Design review of the part built by this model. Coordinates are the model's own, in mm. Coordinates: 2 decimals unless noted, no trailing zeros. Write each loop counter-clockwise with the first axis right and the second up, starting at its lowest first coordinate (ties: lowest second). Pieces come first, ordered by that corner, then holes. Notation, with made-up numbers: (6.5, -24.75) - (28.5, -24.75) arc R29 ccw to (28.5, 13.25) - close; hole circle Ø3 at (79, 51.5). An arc over 180 degrees is marked (long way). One line per item, written item: value.
from build123d import *

# Parameters (mm, degrees)
EXTRUDE_THIN1_DEPTH = 0.53
SKETCH2_R           = 1.151524856
CUT_EXTRUDE1_DEPTH  = 16.607776908


with BuildPart() as part:
    # Sketch1 → Extrude-Thin1 (new body)
    with BuildSketch(Plane(origin=(0, 0, 0), x_dir=(1, 0, 0), z_dir=(0, 1, 0))):
        with BuildLine():
            ThreePointArc((9.712852175, 5.226987912), (-10.721135618, -2.591939635), (11.027949059, -0.212695892))
            Line((11.027949059, -0.212695892), (9.378255864, -0.180878284))
            ThreePointArc((9.378255864, -0.180878284), (-9.117339265, -2.204206144), (8.259886981, 4.445072223))
            Line((8.259886981, 4.445072223), (9.712852175, 5.226987912))
        make_face()
    extrude(amount=EXTRUDE_THIN1_DEPTH)

    # Sketch2 → Cut-Extrude1 (cut, through all)
    with BuildSketch(Plane(origin=(0, 0, 0), x_dir=(1, 0, 0), z_dir=(0, 1, 0))):
        with Locations((8.259886981, 4.445072223)):
            Circle(SKETCH2_R)
    extrude(amount=CUT_EXTRUDE1_DEPTH, mode=Mode.SUBTRACT)


solid = part.part
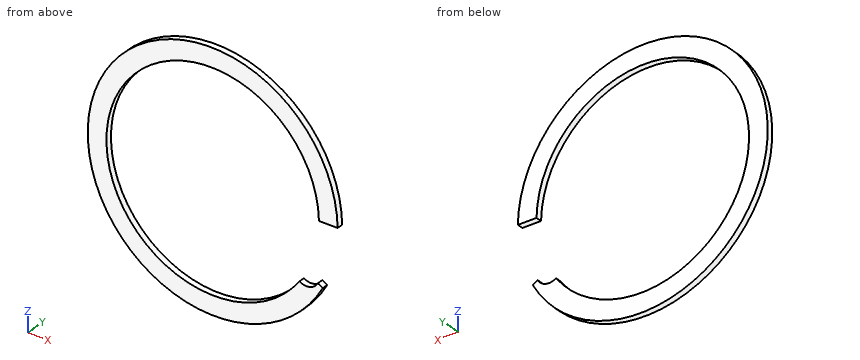
1. Wall thickness on line 1 along Z through (x, y) = (0, 0.45); line 2 along X through (y, z) = (0.3, 0); line 3 along Z through (x, y) = (7, 0.2): over which ranges is each line inside the solid? List them lowest first.
Answer block:
line 1: z = -11.03 to -9.38, 9.38 to 11.03
line 2: x = -11.03 to -9.38
line 3: z = -8.52 to -6.24, 6.24 to 8.52
2. Consider section A-A, the plane x = 0. Write out the cut boundary in (y, z), then the cut area to 3 significant figures.
Answer block:
outline: (0, -11.03) - (0.53, -11.03) - (0.53, -9.38) - (0, -9.38) - close; (0, 9.38) - (0.53, 9.38) - (0.53, 11.03) - (0, 11.03) - close
area: 1.75 mm^2
3. Consider section D-D, the plane z = -1.5. Write out the cut boundary in (x, y).
Answer block:
outline: (-10.93, 0) - (-9.26, 0) - (-9.26, 0.53) - (-10.93, 0.53) - close
4. Consider section C-C, the plane x = -5. Write out the cut boundary in (y, z), then the cut area to 3 significant figures.
Answer block:
outline: (0, -9.83) - (0.53, -9.83) - (0.53, -7.94) - (0, -7.94) - close; (0, 7.94) - (0.53, 7.94) - (0.53, 9.83) - (0, 9.83) - close
area: 2.01 mm^2
5. Consider section B-B, the plane y = 0.4. Write out the cut boundary in (x, z), then the cut area to 3 significant figures.
Answer block:
outline: (7.65, -5.42) arc R9.38 cw (long way) to (9.38, 0.18) - (11.03, 0.21) arc R11.03 ccw (long way) to (9.71, -5.23) - (9.27, -4.99) arc R1.15 cw to start
area: 96.1 mm^2
